Read the model definition and answer for the solid it produces. Units are mm, in the model's axes. Face numbers are marked on the shaded views. A direction names the side the tool comes from. Coordinates: 2 decimals unless noted, no trailing zeros. Loops run counter-clockwise (first coordinate to the right, second up) from the corner with the lowest first, then second, coordinate; pieces in that order, holes last. Notation, with made-up numbers: M 66.5,35.5 L 119.5,35.5 A14 ccw 119.5,44.5 Z; hole C -22.75,41 d1. An arc over 180 degrees is marked long. One line per item, written item: value. Start each with the question number.
1. Consider probe 1 along X at (y, z) = (11.43, 2.5); probe 2 along X at (y, z) = (12, -4.5); probe 3 along Y at (x, z) = (19.5, -9). Determine where each line is inside the solid, lowest interval first.
2. Determine the mould class of the marked faces 4, 5 and 6 for opening direction X: +X half, -X half, draft (parallel to the pull), parting line (faces both ways), or undercut.
3. The part is cut by section D-D (y = 26). Write down the section's boundary in (x, z), then the cut area to 3 significant figures.
4. The part is cut by section B-B (y = 11.43). Write down the section's boundary in (x, z).
5. For the marked faces 1, 2 and 3, determine the directions among +Z, -Z, +X, -X, +Y, -Y from which every point of the face is accessible in a straight line to the end or side of a thin tool.
6. The part is cut by section A-A (z = -7). Write down the section's boundary in (x, y), then the cut area to 3 significant figures.
7. Flat-ended cylindrical pins translate along their axes: pin 1 (10 mm diameter, centred on x = 46, y = 10.5, fed in from -Z); pin 2 (12.5 mm diameter, centred on x = 41.5, y = 13.5, fed in from +Z); pin 3 (8 mm diameter, centred on x = 11.5, z = -25.5, fed in from -Y). Find the tip coordinate at first contact, or state that the pin passes through.
8. The part is cut by section C-C (x = 17.5). Write down the section's boundary in (y, z) (3 decimals).
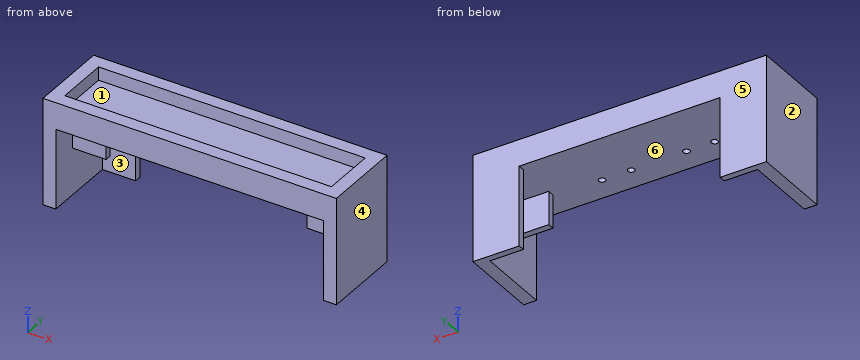
```python
from build123d import *

# Parameters (mm, degrees)
F0_W     = 139.7
F0_H     = 38.1
F1_DEPTH = 6.35
F2_W     = 15.875
F2_H     = 3.1242
F3_DEPTH = 38.1
F4_DEPTH = 15.875
F5_DEPTH = 15.875
F6_W     = 139.7
F6_H     = 38.1
F6_W_2   = 127
F6_H_2   = 25.4
F7_DEPTH = 6.35
F8_R     = 1.5875
F9_DEPTH = 25.4


with BuildPart() as f1:
    # F0 (on Top) → F1 (new body)
    with BuildSketch(Plane.XY):
        with Locations((69.85, 19.05)):
            Rectangle(F0_W, F0_H)
    extrude(amount=F1_DEPTH)

    # F2 (on face) → F3 (join)
    with BuildSketch(Plane(origin=(0, 0, 0), x_dir=(1, 0, 0), z_dir=(0, 0, -1))):
        with Locations((14.0335, -36.5379)):
            Rectangle(F2_W, F2_H)
        Polygon((6.096, 0), (0, 0), (0, -38.1), (6.096, -38.1), (6.096, -34.9758), (6.096, -15.8242), (6.096, -12.7), (6.096, -3.1242), align=None)
        with Locations((125.6665, -36.5379)):
            Rectangle(F2_W, F2_H)
        Polygon((139.7, 0), (133.604, 0), (133.604, -12.7), (133.604, -15.8242), (133.604, -34.9758), (133.604, -38.1), (139.7, -38.1), align=None)
    extrude(amount=F3_DEPTH)

    # F2 (on face) → F4 (join)
    with BuildSketch(Plane(origin=(0, 0, 0), x_dir=(1, 0, 0), z_dir=(0, 0, -1))):
        with Locations((14.0335, -14.2621)):
            Rectangle(F2_W, F2_H)
    extrude(amount=F4_DEPTH)

    # F2 (on face) → F5 (join)
    with BuildSketch(Plane(origin=(0, 0, 0), x_dir=(1, 0, 0), z_dir=(0, 0, -1))):
        with Locations((125.6665, -14.2621)):
            Rectangle(F2_W, F2_H)
    extrude(amount=F5_DEPTH)

    # F6 (on face) → F7 (join)
    with BuildSketch(Plane.XY.offset(6.35)):
        with Locations((69.85, 19.05)):
            Rectangle(F6_W, F6_H)
        with Locations((69.85, 19.05)):
            Rectangle(F6_W_2, F6_H_2, mode=Mode.SUBTRACT)
    extrude(amount=F7_DEPTH)

    # F8 (on face) → F9 (cut)
    with BuildSketch(Plane(origin=(0, 0, 0), x_dir=(1, 0, 0), z_dir=(0, 0, -1))):
        with Locations((41.529, -11.43)):
            Circle(F8_R)
        with Locations((54.8894, -11.43)):
            Circle(F8_R)
        with Locations((81.2292, -11.43)):
            Circle(F8_R)
        with Locations((95.123, -11.43)):
            Circle(F8_R)
    extrude(amount=-F9_DEPTH, mode=Mode.SUBTRACT)


solid = f1.part
```
Answer block:
1. probe 1: x = 0 to 39.94, 43.12 to 53.3, 56.48 to 79.64, 82.82 to 93.54, 96.71 to 139.7
1. probe 2: x = 0 to 6.1, 133.6 to 139.7
1. probe 3: y = 12.7 to 15.82, 34.98 to 38.1
2. face 4: +X half
2. face 5: draft
2. face 6: undercut
3. outline: M 0,-38.1 L 6.1,-38.1 L 6.1,0 L 133.6,0 L 133.6,-38.1 L 139.7,-38.1 L 139.7,12.7 L 133.35,12.7 L 133.35,6.35 L 6.35,6.35 L 6.35,12.7 L 0,12.7 Z
3. area: 1,430 mm2
4. outline: M 0,-38.1 L 6.1,-38.1 L 6.1,0 L 39.94,0 L 39.94,6.35 L 6.35,6.35 L 6.35,12.7 L 0,12.7 Z; M 43.12,0 L 53.3,0 L 53.3,6.35 L 43.12,6.35 Z; M 56.48,0 L 79.64,0 L 79.64,6.35 L 56.48,6.35 Z; M 82.82,0 L 93.54,0 L 93.54,6.35 L 82.82,6.35 Z; M 96.71,0 L 133.6,0 L 133.6,-38.1 L 139.7,-38.1 L 139.7,12.7 L 133.35,12.7 L 133.35,6.35 L 96.71,6.35 Z
5. face 1: +Z
5. face 2: +Z, -Z, -X, +Y, -Y
5. face 3: -Z
6. outline: M 0,0 L 6.1,0 L 6.1,12.7 L 21.97,12.7 L 21.97,15.82 L 6.1,15.82 L 6.1,34.98 L 21.97,34.98 L 21.97,38.1 L 0,38.1 Z; M 117.73,12.7 L 133.6,12.7 L 133.6,0 L 139.7,0 L 139.7,38.1 L 117.73,38.1 L 117.73,34.98 L 133.6,34.98 L 133.6,15.82 L 117.73,15.82 Z
6. area: 663 mm2
7. pin 1: stops at z = 0
7. pin 2: stops at z = 6.35
7. pin 3: stops at y = 34.98
8. outline: M 0,0 L 12.7,0 L 12.7,-15.875 L 15.824,-15.875 L 15.824,0 L 34.976,0 L 34.976,-38.1 L 38.1,-38.1 L 38.1,12.7 L 31.75,12.7 L 31.75,6.35 L 6.35,6.35 L 6.35,12.7 L 0,12.7 Z
